Build history of the part. All positions in model axes, mm. Face numbers are marked on the shaded views. A direction names the side the tool comes from. Round coordinates to 2 decimals unless told otherwise and drop trailing zeros. Write each loop counter-clockwise with the first axis right and the second up, starting at its lowest first coordinate (ties: lowest second). Pieces come first, ordered by that corner, then holes. Notation, with made-up numbers: (-37, 22) -> (8, 22) arc R13 cw to (8, 26) -> close; hole circle Ø5 at (-20.75, -31). An arc over 180 degrees is marked (long way). Answer in a Markdown table with one row per item.
```python
from build123d import *

# Parameters (mm, degrees)
BOSS_EXTRU_1_DEPTH      = 4
ESQUISSE4_W             = 11
ESQUISSE4_H             = 11
BOSS_EXTRU_2_DEPTH      = 3
BOSS_EXTRU_3_DEPTH      = 3
ESQUISSE6_R             = 1.6
ENL_V_MAT_EXTRU_1_DEPTH = 10
ESQUISSE7_R             = 1.6
ENL_V_MAT_EXTRU_2_DEPTH = 10
BOSS_EXTRU_4_DEPTH      = 4
ESQUISSE10_R            = 1.05
ESQUISSE10_R_2          = 1.6
ENL_V_MAT_EXTRU_3_DEPTH = 4
CHANFREIN1_SIZE         = 1
CHANFREIN2_SIZE         = 3
CHANFREIN3_SIZE         = 2


with BuildPart() as part:
    # Esquisse2 → Boss.-Extru.1 (new body)
    with BuildSketch(Plane(origin=(0, 0, 0), x_dir=(1, 0, 0), z_dir=(0, 1, 0))):
        Polygon((17.5, 0), (17.5, 11.5), (-17.5, 11.5), (-17.5, 0), (-17.5, -11.5), (17.5, -11.5), align=None)
    extrude(amount=BOSS_EXTRU_1_DEPTH)

    # Esquisse4 → Boss.-Extru.2 (add)
    with BuildSketch(Plane.XY.offset(11.5)):
        with Locations((12, 7.750794337)):
            Rectangle(ESQUISSE4_W, ESQUISSE4_H)
    extrude(amount=-BOSS_EXTRU_2_DEPTH)

    # Esquisse5 → Boss.-Extru.3 (add)
    with BuildSketch(Plane(origin=(0, 0, -11.5), x_dir=(-1, 0, 0), z_dir=(0, 0, -1))):
        Polygon((-17.5, 2.494257601), (-17.5, 5.399089221), (-6.928293138, 35.966080358), (2.072303922, 35.966080358), (2.072303922, 32.210427233), (-7.684376604, 4), (-7.684376604, 2.494257601), align=None)
    extrude(amount=-BOSS_EXTRU_3_DEPTH)

    # Esquisse6 → Enlèv. mat.-Extru.1 (cut)
    with BuildSketch(Plane.XY.offset(11.5)):
        with Locations((11.802703711, 8.683300858)):
            Circle(ESQUISSE6_R)
    extrude(amount=-ENL_V_MAT_EXTRU_1_DEPTH, mode=Mode.SUBTRACT)

    # Esquisse7 → Enlèv. mat.-Extru.2 (cut)
    with BuildSketch(Plane(origin=(0, 0, -11.5), x_dir=(-1, 0, 0), z_dir=(0, 0, -1))):
        with Locations((-2.967152129, 32.227121405)):
            Circle(ESQUISSE7_R)
    extrude(amount=-ENL_V_MAT_EXTRU_2_DEPTH, mode=Mode.SUBTRACT)

    # Esquisse8 → Boss.-Extru.4 (add)
    with BuildSketch(Plane.XZ):
        Polygon((4.598369828, -11.5), (0.61743287, -16.416755672), (-25.041628639, -16.416755672), (-25.041628639, 16.416755672), (0.61743287, 16.416755672), (4.598369828, 11.5), align=None)
    extrude(amount=-BOSS_EXTRU_4_DEPTH)

    # Esquisse10 → Enlèv. mat.-Extru.3 (cut)
    with BuildSketch(Plane(origin=(0, 4, 0), x_dir=(1, 0, 0), z_dir=(0, 1, 0))):
        with Locations(Location((-6.665623396, -13.88650623, 0), (0, 0, 270))):
            Circle(ESQUISSE10_R)
        with Locations(Location((-6.665623396, 13.88650623, 0), (0, 0, 270))):
            Circle(ESQUISSE10_R)
        with Locations(Location((-19.541628639, 8.216755672, 0), (0, 0, 270))):
            Circle(ESQUISSE10_R_2)
        with Locations(Location((-19.541628639, -8.216755672, 0), (0, 0, 270))):
            Circle(ESQUISSE10_R_2)
        Polygon((-13.015623396, -11.622936602), (-13.015623396, 11.622936602), (-0.315623396, 11.55), (-0.315623396, -11.55), align=None)
    extrude(amount=-ENL_V_MAT_EXTRU_3_DEPTH, mode=Mode.SUBTRACT)

    # Chanfrein1
    chanfrein1_edges = [part.edges().sort_by_distance(p)[0] for p in [
        (17.5, 0, 0),
    ]]
    chamfer(chanfrein1_edges, length=CHANFREIN1_SIZE)

    # Chanfrein2
    chanfrein2_edges = [part.edges().sort_by_distance(p)[0] for p in [
        (-25.041628639, 2, -16.416755672),
        (-25.041628639, 2, 16.416755672),
    ]]
    chamfer(chanfrein2_edges, length=CHANFREIN2_SIZE)

    # Chanfrein3
    chanfrein3_edges = [part.edges().sort_by_distance(p)[0] for p in [
        (6.5, 13.250794337, 10),
        (17.5, 13.250794337, 10),
    ]]
    chamfer(chanfrein3_edges, length=CHANFREIN3_SIZE)


solid = part.part
```
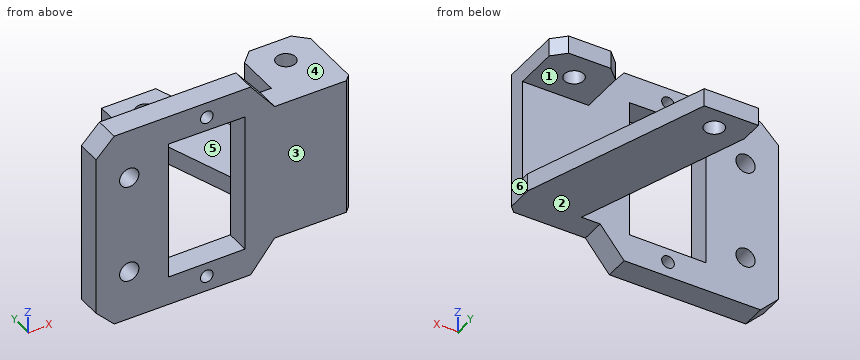
Q1. Wall check: line 1 (Z direction, x = 15.5, y = 10); line 2 (Z direction, x = 4.5, y = 17); line 3 (Y direction, x = 6, z = 3.5). Give the ranges that are in metal, low to high. Write a range as [from, to].
A:
| item | result |
|---|---|
| line 1 | [-11.5, -8.5], [8.5, 11.5] |
| line 2 | [-11.5, -8.5] |
| line 3 | [0, 4] |
Q2. Saw through at C-C on x = -4. Write the cut outline in (y, z).
A:
| item | result |
|---|---|
| outline | (0, -16.42) -> (4, -16.42) -> (4, -11.57) -> (0, -11.57) -> close; (0, 11.57) -> (4, 11.57) -> (4, 16.42) -> (0, 16.42) -> close |
Q3. Which spindle directions (+Z, -Z, +X, -X, +Y, -Y) get a long thin tool onto all of the face, cutting with end or side? Do the marked faces 4, 5 and 6. Say none if no direction does.
A:
| item | result |
|---|---|
| face 4 | +Z, +X, +Y, -Y |
| face 5 | +X, -X, +Y |
| face 6 | +Z, -Z, +X, +Y, -Y |
Q4. Saw through at D-D on y = 12. Write the cut outline in (x, z).
A:
| item | result |
|---|---|
| outline | (4.92, -11.5) -> (15.22, -11.5) -> (15.22, -8.5) -> (4.92, -8.5) -> close; (7.25, 8.5) -> (16.75, 8.5) -> (16.75, 11.5) -> (7.25, 11.5) -> close |
Q5. Saw through at A-A on z = 0. Write the cut outline in (x, y), plus the area to 3 significant figures.
A:
| item | result |
|---|---|
| outline | (-25.04, 0) -> (-13.02, 0) -> (-13.02, 4) -> (-25.04, 4) -> close; (-0.32, 0) -> (16.5, 0) -> (17.5, 1) -> (17.5, 4) -> (-0.32, 4) -> close |
| area | 119 mm² |
Q6. Two-plate mould, pull along Z, no slides. Class the marked faces 1, 2 and 3: released by +Z, released by -Z, zero draft, split by the parting line, or undercut.
A:
| item | result |
|---|---|
| face 1 | undercut |
| face 2 | released by -Z |
| face 3 | zero draft |
Q7. Drop flat-ended pins along their axis: P1, Ø4, axis at x = 9, z = 5.5, coming from the +Y side; P2, Ø3.5, axis at y = 34, z = -9.5, coming from the -X side; P3, Ø2, axis at x = 2, y = 5.5, coming from the +Z side; P4, Ø7.5, axis at x = 13, y = 8.5, coming from the -Z side. Give the stop position or say it passes through.
A:
| item | result |
|---|---|
| P1 | y = 4 |
| P2 | x = -2.07 |
| P3 | through |
| P4 | z = -11.5 |
Q8. Saw through at B-B on z = 10.5. Write the cut outline in (x, y), plus the area to 3 significant figures.
A:
| item | result |
|---|---|
| outline | (-25.04, 0) -> (-13.02, 0) -> (-13.02, 4) -> (-25.04, 4) -> close; (-0.32, 0) -> (16.5, 0) -> (17.5, 1) -> (17.5, 11.25) -> (15.5, 13.25) -> (8.5, 13.25) -> (6.5, 11.25) -> (6.5, 4) -> (-0.32, 4) -> close; hole circle Ø3.2 at (11.8, 8.68) |
| area | 209 mm² |
